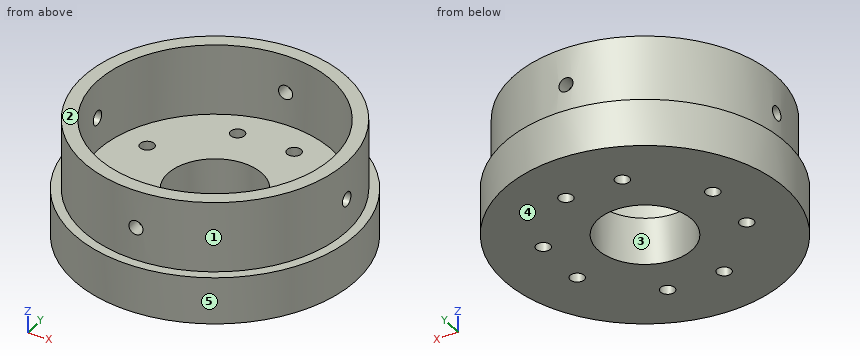
```python
from build123d import *

# Parameters (mm, degrees)
SKETCH_1_R               = 30
EXTRUDE_1_DEPTH          = 10
SKETCH_2_R               = 28
SKETCH_2_R_2             = 25
EXTRUDE_2_DEPTH          = 15
CUT_EXTRUDE_1_DEPTH      = 72.589105316
CUT_EXTRUDE_1_DEPTH_BACK = 72.589105316
SKETCH_3_R               = 1.5
CUT_EXTRUDE_2_DEPTH      = 70.094138717
CUT_EXTRUDE_2_DEPTH_BACK = 70.094138717
SKETCH_4_R               = 1.5
SKETCH_5_R               = 1.5
CUT_EXTRUDE_3_DEPTH      = 15
SKETCH_6_R               = 10
CUT_EXTRUDE_4_DEPTH      = 10


with BuildPart() as part:
    # 스케치1 → 보스-돌출1 (new body)
    with BuildSketch(Plane.XY):
        Circle(SKETCH_1_R)
    extrude(amount=EXTRUDE_1_DEPTH)

    # 스케치2 → 보스-돌출2 (add)
    with BuildSketch(Plane.XY.offset(10)):
        Circle(SKETCH_2_R)
        Circle(SKETCH_2_R_2, mode=Mode.SUBTRACT)
    extrude(amount=EXTRUDE_2_DEPTH)

    # 스케치3 → 컷-돌출1 (cut, two sides: drawn at the far end of the back side and taken through both)
    with BuildSketch(Plane(origin=(0, 30, 0), x_dir=(1, 0, 0), z_dir=(0, 1, 0)).offset(-CUT_EXTRUDE_1_DEPTH_BACK)):
        with Locations(Location((0, -17, 0), (0, 0, 180))):
            Circle(SKETCH_3_R)
    extrude(amount=CUT_EXTRUDE_1_DEPTH + CUT_EXTRUDE_1_DEPTH_BACK, mode=Mode.SUBTRACT)

    # 스케치4 → 컷-돌출2 (cut, two sides: drawn at the far end of the back side and taken through both)
    with BuildSketch(Plane.ZY.offset(27).offset(-CUT_EXTRUDE_2_DEPTH_BACK)):
        with Locations(Location((17, 0, 0), (0, 0, 270))):
            Circle(SKETCH_4_R)
    extrude(amount=CUT_EXTRUDE_2_DEPTH + CUT_EXTRUDE_2_DEPTH_BACK, mode=Mode.SUBTRACT)

    # 스케치5 → 컷-돌출3 (cut)
    with BuildSketch(Plane(origin=(0, 0, 0), x_dir=(-1, 0, 0), z_dir=(0, 0, -1))):
        with Locations((-6, -18)):
            Circle(SKETCH_5_R)
        with Locations((6, -18)):
            Circle(SKETCH_5_R)
        with Locations((18, -6)):
            Circle(SKETCH_5_R)
        with Locations((18, 6)):
            Circle(SKETCH_5_R)
        with Locations((6, 18)):
            Circle(SKETCH_5_R)
        with Locations((-6, 18)):
            Circle(SKETCH_5_R)
        with Locations((-18, 6)):
            Circle(SKETCH_5_R)
        with Locations((-18, -6)):
            Circle(SKETCH_5_R)
    extrude(amount=-CUT_EXTRUDE_3_DEPTH, mode=Mode.SUBTRACT)

    # 스케치6 → 컷-돌출4 (cut)
    with BuildSketch(Plane(origin=(0, 0, 0), x_dir=(-1, 0, 0), z_dir=(0, 0, -1))):
        Circle(SKETCH_6_R)
    extrude(amount=-CUT_EXTRUDE_4_DEPTH, mode=Mode.SUBTRACT)


solid = part.part
```
Here's how the part is built. I have some questions about the finished solid (model axes, mm). Face numbers are marked on the shaded views. A direction names the side the tool comes from. Give positions to 0.01 mm unless a question says otherwise; leave off trailing zeros. Loops run counter-clockwise (first coordinate to the right, second up) from the corner with the lowest first, then second, coordinate; pieces in that order, holes last. Notation, with made-up numbers: M -17.75,28.5 L 14.25,28.5 A29 cw 14.25,49.5 Z; hole C -13.75,73 d8. An arc over 180 degrees is marked long. Return JSON: item names as keys, results as strings.
Item 1: Thinking about a two-plate mould opening in Y: for the marked faces 3, 4 and 5, which applies, released by +Y, released by -Y, zero draft, split by the parting line, or undercut?
A:
{"face 3": "undercut", "face 4": "zero draft", "face 5": "split by the parting line"}
Item 2: Imagine slicing it at B-B on z = 2.25. State how many separate pieces and enclosed holes the cut face has, then the cut area to 3 significant figures.
A:
{"separate pieces": "1", "enclosed holes": "9", "area": "2,460 mm^2"}
Item 3: Please list where these lines run through material, in increasing order: line 1 (Y direction, x = 0, z = 20.25); line 2 (Z direction, x = 0, y = 26); line 3 (Y direction, x = -18, z = 2.75).
A:
{"line 1": "y = -28 to -25, 25 to 28", "line 2": "z = 0 to 15.5, 18.5 to 25", "line 3": "y = -24 to -7.5, -4.5 to 4.5, 7.5 to 24"}
Item 4: On a 3-axis mill with a long thin cutter (end or side, diameter ignored), from which of +Z, -Z, +X, -X, +Y, -Y can I reach the whole of each face in a straight line? I mean the marked faces 1 and 2. Say none if no direction works.
A:
{"face 1": "+Z", "face 2": "+Z, +X, -X, +Y, -Y"}
Item 5: Imagine slicing it at A-A on y = 0. List the corners of the cut face in (x, z) for me.
A:
{"outline": "M -30,0 L -10,0 L -10,10 L -25,10 L -25,15.5 L -28,15.5 L -28,10 L -30,10 Z; M -28,18.5 L -25,18.5 L -25,25 L -28,25 Z; M 10,0 L 30,0 L 30,10 L 28,10 L 28,15.5 L 25,15.5 L 25,10 L 10,10 Z; M 25,18.5 L 28,18.5 L 28,25 L 25,25 Z"}
Item 6: Imagine slicing it at D-D on y = -18. List the corners of the cut face in (x, z) for me.
A:
{"outline": "M -24,0 L -7.5,0 L -7.5,10 L -17.35,10 L -17.35,25 L -21.45,25 L -21.45,10 L -24,10 Z; M -4.5,0 L 4.5,0 L 4.5,10 L -4.5,10 Z; M 7.5,0 L 24,0 L 24,10 L 21.45,10 L 21.45,25 L 17.35,25 L 17.35,10 L 7.5,10 Z"}
Item 7: Imagine slicing it at C-C on x = -3. List the corners of the cut face in (y, z) for me.
A:
{"outline": "M -29.85,0 L -9.54,0 L -9.54,10 L -24.82,10 L -24.82,25 L -27.84,25 L -27.84,10 L -29.85,10 Z; M 9.54,0 L 29.85,0 L 29.85,10 L 27.84,10 L 27.84,25 L 24.82,25 L 24.82,10 L 9.54,10 Z"}
Item 8: I'm going to push flat-ended pins straight in: pin 1 Ø1 at (x, z) = (-6.5, 8.5) entering from -Y; pin 2 Ø4 at (y, z) = (-12.5, 17) entering from -X; pin 3 Ø25 at (x, y) = (9.5, -1.5) entering from +Z; pin 4 Ø1.8 at (x, z) = (0, 17) entering from +Y. Where does each tip first touch, or does it pass through?
A:
{"pin 1": "stops at y = -29.39", "pin 2": "stops at x = -25.96", "pin 3": "stops at z = 10", "pin 4": "passes through"}
